Read the model definition and answer for the solid it produces. Units are mm, in the model's axes. A direction names the side the tool comes from. Coordinates: 2 decimals unless noted, no trailing zeros. Loops run counter-clockwise (first coordinate to the right, second up) from the corner with the lowest first, then second, coordinate; pieces in that order, holes last.
from build123d import *

# Parameters (mm, degrees)
SKETCH1_R           = 3.175
BOSS_EXTRUDE1_DEPTH = 3.175
SKETCH2_R           = 11.049
SKETCH2_R_2         = 15.875
SKETCH2_R_3         = 1.27
CUT_EXTRUDE1_DEPTH  = 202.930998425
SKETCH3_W           = 38.1
SKETCH3_H           = 6.35
SKETCH3_W_2         = 88.9
CUT_EXTRUDE4_DEPTH  = 202.930998425
CUT_EXTRUDE5_DEPTH  = 202.930998425


with BuildPart() as part:
    # Sketch1 → Boss-Extrude1 (new, symmetric)
    with BuildSketch(Plane.XY):
        with BuildLine():
            Line((-145.783553311, 66.675), (145.783553311, 66.675))
            ThreePointArc((145.783553311, 66.675), (147.900219978, 66.497368874), (149.957676269, 65.969444444))
            ThreePointArc((149.957676269, 65.969444444), (172.789871953, 52.74760778), (189.088888889, 31.999880883))
            ThreePointArc((189.088888889, 31.999880883), (190.142181511, 29.17513943), (190.5, 26.181720723))
            Line((190.5, 26.181720723), (190.5, -22.225))
            ThreePointArc((190.5, -22.225), (186.780256121, -31.205256121), (177.8, -34.925))
            Line((177.8, -34.925), (-177.8, -34.925))
            ThreePointArc((-177.8, -34.925), (-186.780256121, -31.205256121), (-190.5, -22.225))
            Line((-190.5, -22.225), (-190.5, 26.181720723))
            ThreePointArc((-190.5, 26.181720723), (-190.142181511, 29.17513943), (-189.088888889, 31.999880883))
            ThreePointArc((-189.088888889, 31.999880883), (-172.789871953, 52.74760778), (-149.957676269, 65.969444444))
            ThreePointArc((-149.957676269, 65.969444444), (-147.900219978, 66.497368874), (-145.783553311, 66.675))
        make_face()
        with Locations((-127, 0)):
            Circle(SKETCH1_R, mode=Mode.SUBTRACT)
        with Locations((127, 0)):
            Circle(SKETCH1_R, mode=Mode.SUBTRACT)
    extrude(amount=BOSS_EXTRUDE1_DEPTH, both=True)

    # Sketch2 → Cut-Extrude1 (cut, through all)
    with BuildSketch(Plane.XY.offset(3.175)):
        with Locations((-127, 0)):
            Circle(SKETCH2_R)
        with Locations((-155.575, 0)):
            Circle(SKETCH2_R_2)
        with Locations((-155.575, 23.8125)):
            Circle(SKETCH2_R_3)
        with Locations((-138.737019773, 16.837980227)):
            Circle(SKETCH2_R_3)
        with Locations((-138.737019773, -16.837980227)):
            Circle(SKETCH2_R_3)
        with Locations((-155.575, -23.8125)):
            Circle(SKETCH2_R_3)
        with Locations((-172.412980227, -16.837980227)):
            Circle(SKETCH2_R_3)
        with Locations((-179.3875, 0)):
            Circle(SKETCH2_R_3)
        with Locations((-172.412980227, 16.837980227)):
            Circle(SKETCH2_R_3)
        with Locations((-127, 15.875)):
            Circle(SKETCH2_R_3)
        with Locations((-115.774679849, 11.225320151)):
            Circle(SKETCH2_R_3)
        with Locations((-111.125, 0)):
            Circle(SKETCH2_R_3)
        with Locations((-115.774679849, -11.225320151)):
            Circle(SKETCH2_R_3)
        with Locations((-127, -15.875)):
            Circle(SKETCH2_R_3)
        with Locations((-138.225320151, -11.225320151)):
            Circle(SKETCH2_R_3)
        with Locations(Location((138.225320151, 11.225320151, 0), (0, 0, 180))):
            Circle(SKETCH2_R_3)
        with Locations((-138.225320151, 11.225320151)):
            Circle(SKETCH2_R_3)
        with Locations(Location((138.225320151, -11.225320151, 0), (0, 0, 180))):
            Circle(SKETCH2_R_3)
        with Locations(Location((127, -15.875, 0), (0, 0, 180))):
            Circle(SKETCH2_R_3)
        with Locations(Location((115.774679849, -11.225320151, 0), (0, 0, 180))):
            Circle(SKETCH2_R_3)
        with Locations(Location((111.125, 0, 0), (0, 0, 180))):
            Circle(SKETCH2_R_3)
        with Locations(Location((115.774679849, 11.225320151, 0), (0, 0, 180))):
            Circle(SKETCH2_R_3)
        with Locations(Location((127, 15.875, 0), (0, 0, 180))):
            Circle(SKETCH2_R_3)
        with Locations(Location((172.412980227, 16.837980227, 0), (0, 0, 180))):
            Circle(SKETCH2_R_3)
        with Locations(Location((179.3875, 0, 0), (0, 0, 180))):
            Circle(SKETCH2_R_3)
        with Locations(Location((172.412980227, -16.837980227, 0), (0, 0, 180))):
            Circle(SKETCH2_R_3)
        with Locations(Location((155.575, -23.8125, 0), (0, 0, 180))):
            Circle(SKETCH2_R_3)
        with Locations(Location((138.737019773, -16.837980227, 0), (0, 0, 180))):
            Circle(SKETCH2_R_3)
        with Locations(Location((138.737019773, 16.837980227, 0), (0, 0, 180))):
            Circle(SKETCH2_R_3)
        with Locations(Location((155.575, 23.8125, 0), (0, 0, 180))):
            Circle(SKETCH2_R_3)
        with Locations(Location((155.575, 0, 0), (0, 0, 180))):
            Circle(SKETCH2_R_2)
        with Locations(Location((127, 0, 0), (0, 0, 180))):
            Circle(SKETCH2_R)
    extrude(amount=-CUT_EXTRUDE1_DEPTH, mode=Mode.SUBTRACT)

    # Sketch3 → Cut-Extrude4 (cut, through all)
    with BuildSketch(Plane.XY.offset(3.175)):
        with Locations((-120.383553311, 63.5)):
            Rectangle(SKETCH3_W, SKETCH3_H)
        with Locations((120.383553311, 63.5)):
            Rectangle(SKETCH3_W, SKETCH3_H)
        with Locations((0, 63.5)):
            Rectangle(SKETCH3_W_2, SKETCH3_H)
    extrude(amount=-CUT_EXTRUDE4_DEPTH, mode=Mode.SUBTRACT)

    # Sketch4 → Cut-Extrude5 (cut, through all)
    with BuildSketch(Plane.XY.offset(3.175)):
        with BuildLine():
            Line((-63.5, 41.275), (63.5, 41.275))
            ThreePointArc((63.5, 41.275), (72.480256121, 37.555256121), (76.2, 28.575))
            Line((76.2, 28.575), (76.2, -3.175))
            ThreePointArc((76.2, -3.175), (72.480256121, -12.155256121), (63.5, -15.875))
            Line((63.5, -15.875), (-63.5, -15.875))
            ThreePointArc((-63.5, -15.875), (-72.480256121, -12.155256121), (-76.2, -3.175))
            Line((-76.2, -3.175), (-76.2, 28.575))
            ThreePointArc((-76.2, 28.575), (-72.480256121, 37.555256121), (-63.5, 41.275))
        make_face()
    extrude(amount=-CUT_EXTRUDE5_DEPTH, mode=Mode.SUBTRACT)


solid = part.part
Q1. A cutting plane is placed at A-A (y = 49.5). Give the vertices of the cut face in (x, z) (3 decimals), then the cut area to 3 significant figures.
Findings below:
outline: (-176.283, -3.175) - (176.283, -3.175) - (176.283, 3.175) - (-176.283, 3.175) - close
area: 2,240 mm2
Q2. A cutting plane is placed at B-B (z = 0.25). Count the separate pieces of the cut face and the enclosed holes in it, then the cut area to 3 significant figures.
Findings below:
separate pieces: 1
enclosed holes: 33
area: 25,400 mm2
Q3. A flat-ended cylindrical pin translates along its axis: pin 1 Ø1.9 at (x, z) = (124, -1) entering from +Y (3 decimals). Find the tip coordinate at first contact, or state that the pin passes through.
Findings below:
pin 1: stops at y = 60.325
Q4. Which of the six approach directions +Z, -Z, +X, -X, +Y, -Y give full straight-line access (tool end or side, diameter ignored) to faces 4 (the face through (3, -17, 3.175)), 5 (the face through (-72.578, 37.456, 0.044)), 6 (the face through (-1, 60.325, 0))?
Findings below:
face 4: +Z, +X, -X, +Y, -Y
face 5: +Z, -Z
face 6: +Z, -Z, +Y
Q5. Determine the mould class of faces 1 (the face through (-44.45, 63, 0)), 2 (the face through (2, -34.925, 0)), 3 (the face through (1, -15.875, 0)) for opening direction Y: +Y half, -Y half, draft (parallel to the pull), parting line (faces both ways), or undercut.
Findings below:
face 1: draft
face 2: -Y half
face 3: undercut
Q6. Straight lines are drawn through the part: probe 1 along Y at (x, z) = (127, -1) (3 decimals); probe 2 along Y at (x, z) = (-33, -1) (3 decimals); probe 3 along X at (y, z) = (27, 0). For each, find the intervals that lie inside material, in ascending order.
Findings below:
probe 1: y = -34.925 to -17.145, -14.605 to -11.049, 11.049 to 14.605, 17.145 to 60.325
probe 2: y = -34.925 to -15.875, 41.275 to 60.325
probe 3: x = -190.47 to -76.2, 76.2 to 190.47
